Part model, mm, in its own coordinate system. Coordinates: 2 decimals unless noted, no trailing zeros. Order: outer loops, then holes, each group sorted by start corner. A loop starts at its lowest first (then second) coordinate and runs counter-clockwise, first axis right, second up.
from build123d import *

# Parameters (mm, degrees)
BOSS_EXTRUDE1_START     = 25
SKETCH1_W               = 3
SKETCH1_H               = 40
BOSS_EXTRUDE1_DEPTH     = 8
BOSS_EXTRUDE2_START     = 32.5
SKETCH2_W               = 3
SKETCH2_H               = 9.25
SKETCH2_H_2             = 8.5
BOSS_EXTRUDE2_DEPTH     = 32.5
BOSS_EXTRUDE3_START     = 25
SKETCH3_W               = 8
SKETCH3_H               = 4.5
BOSS_EXTRUDE3_DEPTH     = 3
BOSS_EXTRUDE4_START     = 22
SKETCH4_W               = 3
SKETCH4_H               = 3.9
BOSS_EXTRUDE4_DEPTH     = 3
CUT_EXTRUDE1_DEPTH      = 72.175838597
CUT_EXTRUDE1_DEPTH_BACK = 72.175838597
SKETCH5_R               = 1.2
CUT_EXTRUDE2_DEPTH      = 72.175838597
CUT_EXTRUDE2_DEPTH_BACK = 72.175838597
SKETCH6_W               = 1.8
SKETCH6_H               = 1
CUT_EXTRUDE3_DEPTH      = 72.175838597
CUT_EXTRUDE3_DEPTH_BACK = 72.175838597
SKETCH7_W               = 9
SKETCH7_H               = 10.65
SKETCH7_W_2             = 7
SKETCH7_H_2             = 9.9
SKETCH7_W_3             = 13
CUT_EXTRUDE4_DEPTH      = 72.175838597
CUT_EXTRUDE4_DEPTH_BACK = 72.175838597


with BuildPart() as part:
    # Sketch1 → Boss-Extrude1 (new body)
    with BuildSketch(Plane.XY.offset(BOSS_EXTRUDE1_START)):
        with Locations((11.5, 0)):
            Rectangle(SKETCH1_W, SKETCH1_H)
    extrude(amount=BOSS_EXTRUDE1_DEPTH)

    # Sketch2 → Boss-Extrude2 (add)
    with BuildSketch(Plane.XY.offset(BOSS_EXTRUDE2_START)):
        with Locations((11.5, 15.375)):
            Rectangle(SKETCH2_W, SKETCH2_H)
        with Locations((11.5, 5)):
            Rectangle(SKETCH2_W, SKETCH2_H_2)
        with Locations((11.5, -5)):
            Rectangle(SKETCH2_W, SKETCH2_H_2)
        with Locations((11.5, -15.375)):
            Rectangle(SKETCH2_W, SKETCH2_H)
    extrude(amount=BOSS_EXTRUDE2_DEPTH)

    # Sketch3 → Boss-Extrude3 (add)
    with BuildSketch(Plane.XY.offset(BOSS_EXTRUDE3_START)):
        with Locations((17, 17.725)):
            Rectangle(SKETCH3_W, SKETCH3_H)
    extrude(amount=BOSS_EXTRUDE3_DEPTH)

    # Sketch4 → Boss-Extrude4 (add)
    with BuildSketch(Plane.XY.offset(BOSS_EXTRUDE4_START)):
        with Locations((11.5, 17.725)):
            Rectangle(SKETCH4_W, SKETCH4_H)
    extrude(amount=BOSS_EXTRUDE4_DEPTH)

    # Sketch5 → Cut-Extrude1 (cut, two sides: drawn at the far end of the back side and taken through both)
    with BuildSketch(Plane.XY.offset(-CUT_EXTRUDE1_DEPTH_BACK)):
        with Locations((15, 17.725)):
            Circle(SKETCH5_R)
        with Locations((18.5, 17.725)):
            Circle(SKETCH5_R)
    extrude(amount=CUT_EXTRUDE1_DEPTH + CUT_EXTRUDE1_DEPTH_BACK, mode=Mode.SUBTRACT)

    # Sketch6 → Cut-Extrude2 (cut, two sides: drawn at the far end of the back side and taken through both)
    with BuildSketch(Plane(origin=(0, 0, 0), x_dir=(1, 0, 0), z_dir=(0, 1, 0)).offset(-CUT_EXTRUDE2_DEPTH_BACK)):
        with Locations((9.9, -29.5)):
            Rectangle(SKETCH6_W, SKETCH6_H)
        with Locations((9.9, -32)):
            Rectangle(SKETCH6_W, SKETCH6_H)
        with Locations((9.9, -34.5)):
            Rectangle(SKETCH6_W, SKETCH6_H)
        with Locations((9.9, -37)):
            Rectangle(SKETCH6_W, SKETCH6_H)
        with Locations((9.9, -39.5)):
            Rectangle(SKETCH6_W, SKETCH6_H)
        with Locations((9.9, -42)):
            Rectangle(SKETCH6_W, SKETCH6_H)
        with Locations((9.9, -44.5)):
            Rectangle(SKETCH6_W, SKETCH6_H)
        with Locations((9.9, -47)):
            Rectangle(SKETCH6_W, SKETCH6_H)
        with Locations((9.9, -49.5)):
            Rectangle(SKETCH6_W, SKETCH6_H)
        with Locations((9.9, -52)):
            Rectangle(SKETCH6_W, SKETCH6_H)
        with Locations((9.9, -54.5)):
            Rectangle(SKETCH6_W, SKETCH6_H)
        with Locations((9.9, -57)):
            Rectangle(SKETCH6_W, SKETCH6_H)
        with Locations((9.9, -59.5)):
            Rectangle(SKETCH6_W, SKETCH6_H)
    extrude(amount=CUT_EXTRUDE2_DEPTH + CUT_EXTRUDE2_DEPTH_BACK, mode=Mode.SUBTRACT)

    # Sketch7 → Cut-Extrude3 (cut, two sides: drawn at the far end of the back side and taken through both)
    with BuildSketch(Plane(origin=(0, 0, 0), x_dir=(0, 0, -1), z_dir=(1, 0, 0)).offset(-CUT_EXTRUDE3_DEPTH_BACK)):
        with Locations((-65.5, 15.375)):
            Rectangle(SKETCH7_W, SKETCH7_H)
        with Locations((-66.5, -5)):
            Rectangle(SKETCH7_W_2, SKETCH7_H_2)
        with Locations((-63.5, -15.375)):
            Rectangle(SKETCH7_W_3, SKETCH7_H)
    extrude(amount=CUT_EXTRUDE3_DEPTH + CUT_EXTRUDE3_DEPTH_BACK, mode=Mode.SUBTRACT)

    # Sketch8 → Cut-Extrude4 (cut, two sides: drawn at the far end of the back side and taken through both)
    with BuildSketch(Plane(origin=(0, 0, 0), x_dir=(0, 0, -1), z_dir=(1, 0, 0)).offset(-CUT_EXTRUDE4_DEPTH_BACK)):
        Polygon((-58.3, 10.05), (-62, 10.05), (-62, 13.75), align=None)
        Polygon((-58.3, 20.7), (-62, 17), (-62, 20.7), align=None)
        Polygon((-62.3, 0.05), (-66, 0.05), (-66, 3.75), align=None)
        Polygon((-62.3, 9.95), (-66, 6.25), (-66, 9.95), align=None)
        Polygon((-60.3, -9.95), (-64, -9.95), (-64, -6.25), align=None)
        Polygon((-60.3, -0.05), (-64, -3.75), (-64, -0.05), align=None)
        Polygon((-54.3, -20.7), (-58, -20.7), (-58, -17), align=None)
        Polygon((-54.3, -10.05), (-58, -13.75), (-58, -10.05), align=None)
    extrude(amount=CUT_EXTRUDE4_DEPTH + CUT_EXTRUDE4_DEPTH_BACK, mode=Mode.SUBTRACT)


solid = part.part
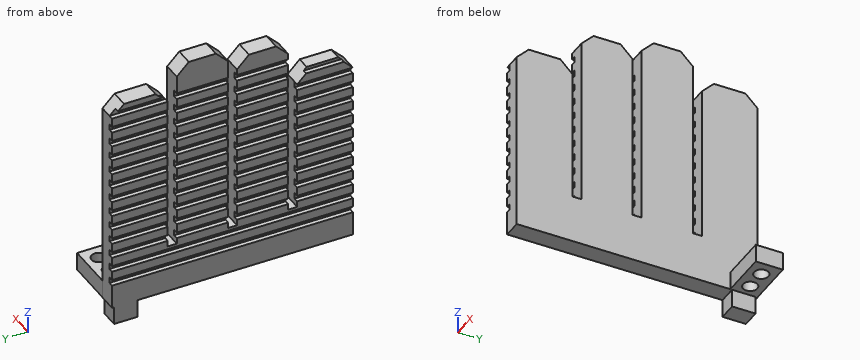
Q1. Cut at C-C on z = 56. Write the cut outline in (x, y), and give its area (4 significant figures).
Results list:
outline: (10, -19) - (13, -19) - (13, -11.75) - (10, -11.75) - close; (10, -9.25) - (13, -9.25) - (13, -0.75) - (10, -0.75) - close; (10, 0.75) - (13, 0.75) - (13, 9.25) - (10, 9.25) - close; (10, 10.75) - (13, 10.75) - (13, 20) - (10, 20) - close
area: 100.5 mm2
Q2. Cut at B-B on x = 18.5. Write the cut outline in (y, z) (3 decimals).
Results list:
outline: (15.475, 25) - (16.525, 25) - (16.525, 28) - (15.475, 28) - close; (18.925, 25) - (19.975, 25) - (19.975, 28) - (18.925, 28) - close
Q3. Wall check: line 1 along Y through (x, z) = (15, 26.3) (3 decimals); line 2 along Y through (x, z) = (10.5, 56); line 3 along X through (y, z) = (-3.5, 38). Give the ranges that are in metal, low to high.
Results list:
line 1: y = 15.475 to 16.525, 18.925 to 19.975
line 2: y = -19 to -11.75, -9.25 to -0.75, 0.75 to 9.25, 10.75 to 20
line 3: x = 10 to 13
Q4. Cut at A-A on z = 48.5. Write the cut outline in (x, y).
Results list:
outline: (10, -20) - (13, -20) - (13, -10.75) - (10, -10.75) - close; (10, -9.25) - (13, -9.25) - (13, -0.75) - (10, -0.75) - close; (10, 0.75) - (13, 0.75) - (13, 9.25) - (10, 9.25) - close; (10, 10.75) - (13, 10.75) - (13, 20) - (10, 20) - close
Q5. Pin check, flat tips, straight feed: pin 1 Ø0.6 at (x, y) = (10.5, -3) entering from +Z; pin 2 Ø0.9 at (x, y) = (10.5, -14) entering from -Z; pin 3 Ø1 at (x, y) = (11.5, 11) entering from +Z. Stop position of each tip, or through.
Results list:
pin 1: stops at z = 63
pin 2: stops at z = 25
pin 3: stops at z = 59.75
